Can you work these out from the drawing? Everything is in mm from the part's minimum corner. A direction names the side the tool comes from. Round coordinates to 2 decimals unless told otherwise and drop trailing zeros. Order: outer loops, then holes, each group sorted by start corner. A loop starts at its lowest first (then second) coordinate and runs counter-clockwise, first axis right, second up. Notation, with made-up numbers: (-21.5, 61.25) - (34.5, 61.25) arc R24 cw to (34.5, 98.25) - close; hole circle Ø6 at (43, 21). An arc over 180 degrees is marked (long way). Write item = value, one per line.
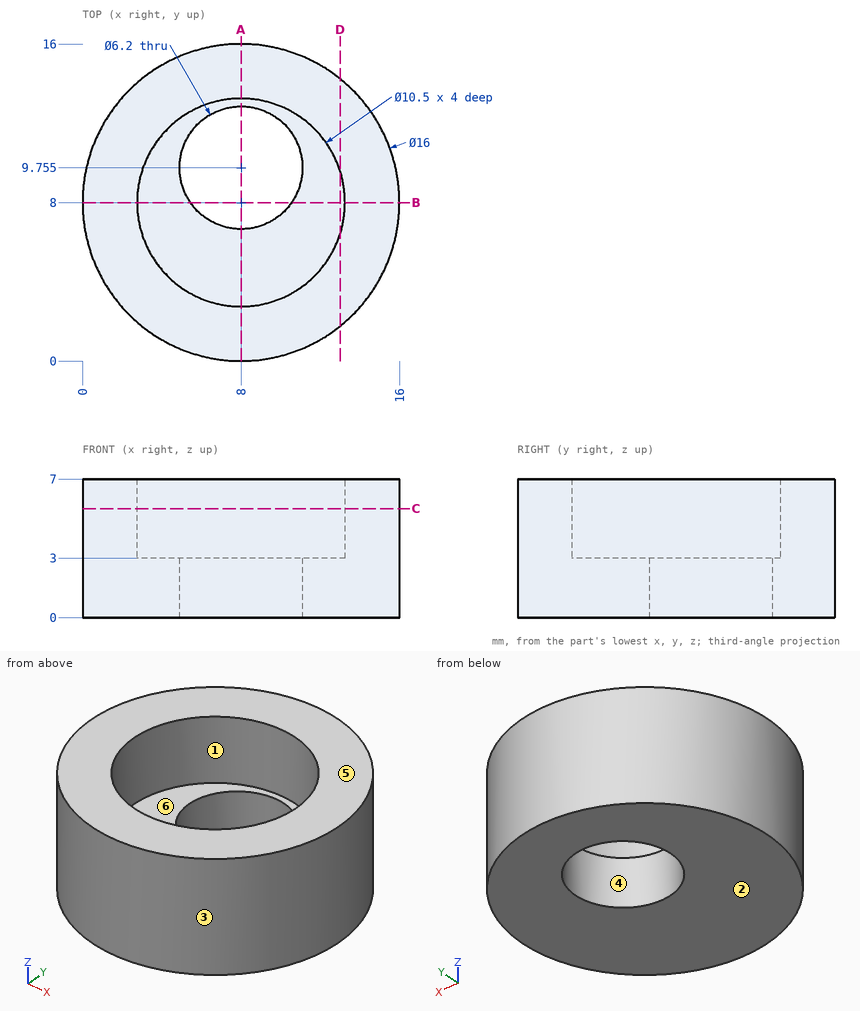
(1) If I drill on line 1 (Y direction, x = 8, z = 1.65) (3 decimals); line 2 (Z direction, x = 5, y = 11.75); line 3 (Y direction, x = 8, z = 5.2), over which ranges is the centre line in solid material (lowest first)? Write a range as from..to.
Computed:
line_1 = 0..6.655, 12.855..16
line_2 = 0..3
line_3 = 0..2.75, 13.25..16
(2) Will these pins go through, and if not, where does the flat tip stop? P1, Ø3, axis at x = 10, y = 10, coming from the +Z side; P2, Ø6.5, axis at x = 8, y = 8, coming from the -Z side; P3, Ø1.5, axis at y = 6, z = 1.5, coming from the -X side; P4, Ø1.5, axis at x = 14, z = 5, coming from the -Y side.
Computed:
P1 = 3
P2 = 0
P3 = 0.1
P4 = 1.96
(3) On a 3-axis mill with a long thin cutter (end or side, diameter ignored), from which of +Z, -Z, +X, -X, +Y, -Y can I reach the whole of each face in a straight line? I mean the marked faces 1 and 2. Say none if no direction works.
Computed:
face_1 = +Z
face_2 = -Z, +X, -X, +Y, -Y
(4) If we section it at C-C (z = 5.5): Write out the boundary of the cut face in (x, y), plus the area to 3 significant figures.
Computed:
outline = circle Ø16 at (8, 8); hole circle Ø10.5 at (8, 8)
area = 114 mm^2
(5) Thinking about a two-plate mould opening in Y: for the marked faces 3, 4, 5 and 6, which applies, +Y half, -Y half, draft (parallel to the pull), parting line (faces both ways), or undercut?
Computed:
face_3 = parting line
face_4 = undercut
face_5 = draft
face_6 = undercut
(6) If we section it at D-D (x = 13): Write out the boundary of the cut face in (y, z) (3 decimals).
Computed:
outline = (1.755, 0) - (14.245, 0) - (14.245, 7) - (9.601, 7) - (9.601, 3) - (6.399, 3) - (6.399, 7) - (1.755, 7) - close
(7) If we section it at B-B (y = 8): Write out the boundary of the cut face in (x, z).
Computed:
outline = (0, 0) - (5.44, 0) - (5.44, 3) - (2.75, 3) - (2.75, 7) - (0, 7) - close; (10.56, 0) - (16, 0) - (16, 7) - (13.25, 7) - (13.25, 3) - (10.56, 3) - close
(8) If we section it at A-A (x = 8): Write out the boundary of the cut face in (y, z) (3 decimals).
Computed:
outline = (0, 0) - (6.655, 0) - (6.655, 3) - (2.75, 3) - (2.75, 7) - (0, 7) - close; (12.855, 0) - (16, 0) - (16, 7) - (13.25, 7) - (13.25, 3) - (12.855, 3) - close
